```python
from build123d import *

# Parameters (mm, degrees)
SKETCH1_W           = 91.948
SKETCH1_H           = 61.468
BOSS_EXTRUDE1_DEPTH = 2.8956
SKETCH2_W           = 33.1216
SKETCH2_H           = 33.1216
BOSS_EXTRUDE2_DEPTH = 5.3848
FILLET1_R           = 2.54


with BuildPart() as part:
    # Sketch1 → Boss-Extrude1 (new body)
    with BuildSketch(Plane(origin=(0, 0, 0), x_dir=(1, 0, 0), z_dir=(0, 1, 0))):
        with Locations((45.974, 30.734)):
            Rectangle(SKETCH1_W, SKETCH1_H)
    extrude(amount=BOSS_EXTRUDE1_DEPTH)

    # Sketch2 → Boss-Extrude2 (add)
    with BuildSketch(Plane.XZ):
        with Locations((16.5608, -30.734)):
            Rectangle(SKETCH2_W, SKETCH2_H)
    extrude(amount=BOSS_EXTRUDE2_DEPTH)

    # Fillet1
    fillet1_edges = [part.edges().sort_by_distance(p)[0] for p in [
        (91.948, 2.8956, -30.734),
        (45.974, 2.8956, -61.468),
        (0, 2.8956, -30.734),
        (45.974, 2.8956, 0),
    ]]
    fillet(fillet1_edges, radius=FILLET1_R)


solid = part.part
```
Geometry check sheet. Reference: the model listing, model coordinates, mm. A direction names the side the tool comes from. Coordinates: 2 decimals unless noted, no trailing zeros. Loops run counter-clockwise (first coordinate to the right, second up) from the corner with the lowest first, then second, coordinate; pieces in that order, holes last. Notation, with made-up numbers: (40, -26) -> (78, -26) arc R20 cw to (78, 11) -> close; hole circle Ø6 at (-30.5, 5.5). An arc over 180 degrees is marked (long way). Put each result on its own line as item: value.
1) Thickness scan on line 1 (Y direction, x = 47, z = -12); line 2 (X direction, y = -4, z = -29); line 3 (Z direction, x = 31, y = -3.75). Record the ranges inside material, lowest first.
Result set:
line 1: y = 0 to 2.9
line 2: x = 0 to 33.12
line 3: z = -47.29 to -14.17
2) Cross-section at B-B on z = -38. Record the boundary of the cut face in (x, y), plus the area to 3 significant figures.
Result set:
outline: (0, -5.38) -> (33.12, -5.38) -> (33.12, 0) -> (91.95, 0) -> (91.95, 0.36) arc R2.54 ccw to (89.41, 2.9) -> (2.54, 2.9) arc R2.54 ccw to (0, 0.36) -> close
area: 442 mm^2
3) Cross-section at D-D on z = -7. Record the boundary of the cut face in (x, y), plus the area to 3 significant figures.
Result set:
outline: (0, 0) -> (91.95, 0) -> (91.95, 0.36) arc R2.54 ccw to (89.41, 2.9) -> (2.54, 2.9) arc R2.54 ccw to (0, 0.36) -> close
area: 263 mm^2
4) Gauge pin test, flat ends, axial feed: pin 1 Ø1.6 at (x, y) = (17, -3) entering from +Z; pin 2 Ø3 at (y, z) = (-1.5, -29) entering from -X; pin 3 Ø4 at (x, z) = (21.5, -53) entering from -Y; pin 4 Ø1.6 at (x, y) = (19, -2.5) entering from -Z. Record the tip position at first contact, or that the pin passes through.
Result set:
pin 1: stops at z = -14.17
pin 2: stops at x = 0
pin 3: stops at y = 0
pin 4: stops at z = -47.29
5) Tool access check on faces 1 (the flat face through (16, -3, -14.173)), 2 (the flat face through (16, -3, -47.295)), 3 (the flat face through (33.122, -3, -31)), 4 (the cylindrical face through (91.184, 2.171, -31.164)). Record the directions out of +Z, -Z, +X, -X, +Y, -Y that give a thin tool (end or side, any length) a straight path to the whole face; none if there is none.
Result set:
face 1: +Z, +X, -X, -Y
face 2: -Z, +X, -X, -Y
face 3: +Z, -Z, +X, -Y
face 4: +Z, -Z, +X, +Y
6) Cross-section at C-C on y = -3.75. Record the boundary of the cut face in (x, z), plus the area to 3 significant figures.
Result set:
outline: (0, -47.29) -> (33.12, -47.29) -> (33.12, -14.17) -> (0, -14.17) -> close
area: 1,100 mm^2
7) Cross-section at A-A on x = 19. Record the boundary of the cut face in (y, z), plus the area to 3 significant figures.
Result set:
outline: (-5.38, -47.29) -> (0, -47.29) -> (0, -61.47) -> (0.36, -61.47) arc R2.54 ccw to (2.9, -58.93) -> (2.9, -2.54) arc R2.54 ccw to (0.36, 0) -> (0, 0) -> (0, -14.17) -> (-5.38, -14.17) -> close
area: 354 mm^2
